Geometry: final body of the model. Coordinates: model frame, mm. A direction names the side the tool comes from. Round coordinates to 2 decimals unless told otherwise and drop trailing zeros. Loops run counter-clockwise (first coordinate to the right, second up) from the corner with the lowest first, then second, coordinate; pieces in that order, holes last. Notation, with made-up numbers: (68.5, -36) - (121.5, -36) arc R34 cw to (121.5, 3) - close; hole circle Ø3 at (-16, 21.25). An arc over 180 degrees is marked (long way). Return JSON: item names as keys, results as strings. Group by question number.
1. Section A-A on x = -65. Return loops of the section in (y, z).
2. Section B-B on z = 65. Return loops of the section in (x, y), and give its area (3 significant figures).
3. Section D-D on z = 0. Return loops of the section in (x, y).
4. Set-up query: faces 1 (the face through (-51.04, -0.99, -27.43)), 2 (the face through (15, 0, 17)). Return all of +Z, -Z, +X, -X, +Y, -Y with unobstructed straight access to the full face (end or side cutting, diameter ignored); none if empty.
5. Section C-C on x = 0. Return loops of the section in (y, z).
6. Material intervals for probe 1 along Z at (x, y) = (-65, -0.4); probe 2 along X at (y, z) = (-0.35, 33); probe 3 along X at (y, z) = (-1.3, 49), sorted ascending.
7. Draft query along Z for faces 3 (the face through (15, -2, 17)), 4 (the face through (-33.96, -0.99, -57.57)). Return one class per face: +Z half, -Z half, draft (parallel to the pull), parting line (faces both ways), or undercut.
from build123d import *

# Parameters (mm, degrees)
SKETCH_W     = 140
SKETCH_H     = 140
SKETCH_R     = 20
PAD_DEPTH    = 2
SKETCH001_R  = 2
POCKET_DEPTH = 2.001


with BuildPart() as part:
    # Sketch → Pad (new body)
    with BuildSketch(Plane.XZ):
        Rectangle(SKETCH_W, SKETCH_H)
        Circle(SKETCH_R, mode=Mode.SUBTRACT)
        Polygon((-42.5, 22.5), (-25.179492, 52.5), (-59.820508, 52.5), align=None, mode=Mode.SUBTRACT)
        Polygon((42.5, -22.5), (25.179492, -52.5), (59.820508, -52.5), align=None, mode=Mode.SUBTRACT)
        Polygon((54.255705, 26.31966), (61.52113, 48.68034), (42.5, 62.5), (23.47887, 48.68034), (30.744295, 26.31966), align=None, mode=Mode.SUBTRACT)
        Polygon((-42.5, -22.5), (-59.820508, -32.5), (-59.820508, -52.5), (-42.5, -62.5), (-25.179492, -52.5), (-25.179492, -32.5), align=None, mode=Mode.SUBTRACT)
    extrude(amount=PAD_DEPTH)

    # Sketch001 (on Face24 of Pad) → Pocket (cut, through all)
    with BuildSketch(Plane.XZ.offset(2)):
        with Locations((-65, 65)):
            Circle(SKETCH001_R)
        with Locations((65, 65)):
            Circle(SKETCH001_R)
        with Locations((65, -65)):
            Circle(SKETCH001_R)
        with Locations((-65, -65)):
            Circle(SKETCH001_R)
    extrude(amount=-POCKET_DEPTH, mode=Mode.SUBTRACT)


solid = part.part
Taken from the geometry:
{
 "1": {"outline": "(-2, -70) - (0, -70) - (0, -67) - (-2, -67) - close; (-2, -63) - (0, -63) - (0, 63) - (-2, 63) - close; (-2, 67) - (0, 67) - (0, 70) - (-2, 70) - close"},
 "2": {"outline": "(-70, -2) - (-67, -2) - (-67, 0) - (-70, 0) - close; (-63, -2) - (63, -2) - (63, 0) - (-63, 0) - close; (67, -2) - (70, -2) - (70, 0) - (67, 0) - close", "area": "264 mm2"},
 "3": {"outline": "(-70, -2) - (-20, -2) - (-20, 0) - (-70, 0) - close; (20, -2) - (70, -2) - (70, 0) - (20, 0) - close"},
 "4": {"face 1": "+Y, -Y", "face 2": "+Z, -Z, +X, -X, +Y"},
 "5": {"outline": "(-2, -70) - (0, -70) - (0, -20) - (-2, -20) - close; (-2, 20) - (0, 20) - (0, 70) - (-2, 70) - close"},
 "6": {"probe 1": "-70 to -67, -63 to 63, 67 to 70", "probe 2": "-70 to -48.56, -36.44 to 28.57, 56.43 to 70", "probe 3": "-70 to -57.8, -27.2 to 23.92, 61.08 to 70"},
 "7": {"face 3": "draft", "face 4": "undercut"}
}
